```python
from build123d import *

# Parameters (mm, degrees)
BOSS_EXTRUDE1_DEPTH     = 3.556
CIRPATTERN1_COUNT       = 15
SKETCH2_W               = 7.954934775
SKETCH2_H               = 1.5875
SKETCH9_R               = 19.84375
SKETCH9_R_2             = 1.5
BOSS_EXTRUDE2_DEPTH     = 1.5875
SKETCH3_R               = 1.74625
CUT_EXTRUDE1_DEPTH      = 6.087499985
CUT_EXTRUDE1_DEPTH_BACK = 6.087499985
CIRPATTERN2_COUNT       = 4
SKETCH12_R              = 3.175
CUT_EXTRUDE2_DEPTH      = 3.175
SKETCH13_R              = 1.525
CUT_EXTRUDE4_DEPTH      = 7.99999997


with BuildPart() as part:
    # Sketch1 → Boss-Extrude1 (new body, symmetric)
    with BuildSketch(Plane(origin=(0, 0, 0), x_dir=(1, 0, 0), z_dir=(0, 1, 0))):
        with BuildLine():
            ThreePointArc((0.866466766, 6.246873729), (0.552789859, 5.752672402), (0, 5.560184675))
            ThreePointArc((0, 5.560184675), (-1.156027397, -5.438681299), (2.261530849, 5.079481453))
            ThreePointArc((2.261530849, 5.079481453), (1.834823997, 5.480167634), (1.749275672, 6.059226903))
            ThreePointArc((1.749275672, 6.059226903), (1.687548707, 6.408986287), (1.409147818, 6.629519254))
            ThreePointArc((1.409147818, 6.629519254), (1.065117112, 6.541288206), (0.866466766, 6.246873729))
        make_face()
    boss_extrude1 = extrude(amount=BOSS_EXTRUDE1_DEPTH, both=True)

    # CirPattern1: Boss-Extrude1 ×15 about axis
    cirpattern1_axis = Axis((0, 0, 0), (0, 1, 0))
    for i in range(1, CIRPATTERN1_COUNT):
        add(boss_extrude1.rotate(cirpattern1_axis, i * 360 / CIRPATTERN1_COUNT))

    # Sketch2 → Revolve3 (revolve)
    with BuildSketch(Plane(origin=(0, 0, 0), x_dir=(0, 0, -1), z_dir=(1, 0, 0))):
        with Locations((3.977467388, 4.293749985)):
            Rectangle(SKETCH2_W, SKETCH2_H)
    revolve3 = revolve(axis=Axis((0, 3.3, 0), (0, -1, 0)))

    # Mirror1: Revolve3 across plane
    add(revolve3.mirror(Plane.ZX))

    # Sketch9 → Boss-Extrude2 (add)
    with BuildSketch(Plane.XZ.offset(5.087499985)):
        Circle(SKETCH9_R)
        Circle(SKETCH9_R_2, mode=Mode.SUBTRACT)
    extrude(amount=-BOSS_EXTRUDE2_DEPTH)

    # Sketch3 → Cut-Extrude1 (cut, two sides)
    with BuildSketch(Plane(origin=(0, 0, 0), x_dir=(1, 0, 0), z_dir=(0, 1, 0))) as cut_extrude1_sk:
        with Locations((-15.5, 0)):
            Circle(SKETCH3_R)
        with Locations((0, 15.5)):
            Circle(SKETCH3_R)
        with Locations((15.5, 0)):
            Circle(SKETCH3_R)
        with Locations((0, -15.5)):
            Circle(SKETCH3_R)
    extrude(amount=CUT_EXTRUDE1_DEPTH, mode=Mode.SUBTRACT)
    extrude(cut_extrude1_sk.sketch, amount=-CUT_EXTRUDE1_DEPTH_BACK, mode=Mode.SUBTRACT)

    # Sketch6 → Cut-Revolve2 (revolve, cut)
    with BuildSketch(Plane.XY):
        Polygon((-11.8678, -3.499999985), (-15.5, -7.132199985), (-15.5, -3.499999985), align=None)
    cut_revolve2 = revolve(axis=Axis((-15.5, -5.087499985, 0), (0, 1, 0)), mode=Mode.SUBTRACT)

    # CirPattern2: Cut-Revolve2 ×4 about axis
    cirpattern2_axis = Axis((0, 0, 0), (0, 1, 0))
    for i in range(1, CIRPATTERN2_COUNT):
        add(cut_revolve2.rotate(cirpattern2_axis, i * 360 / CIRPATTERN2_COUNT), mode=Mode.SUBTRACT)

    # Sketch12 → Cut-Extrude2 (cut)
    with BuildSketch(Plane(origin=(0, 5.087499985, 0), x_dir=(1, 0, 0), z_dir=(0, 1, 0))):
        Circle(SKETCH12_R)
    extrude(amount=-CUT_EXTRUDE2_DEPTH, mode=Mode.SUBTRACT)

    # Sketch13 → Cut-Extrude4 (cut, through all)
    with BuildSketch(Plane(origin=(0, 1.912499985, 0), x_dir=(1, 0, 0), z_dir=(0, 1, 0))):
        Circle(SKETCH13_R)
    extrude(amount=-CUT_EXTRUDE4_DEPTH, mode=Mode.SUBTRACT)


solid = part.part
```
CAD build for the part. Positions are in the model's coordinates, mm. A direction names the side the tool comes from. Give positions to 0.01 mm unless a question says otherwise; leave off trailing zeros. Order: outer loops, then holes, each group sorted by start corner. A loop starts at its lowest first (then second) coordinate and runs counter-clockwise, first axis right, second up.
(1) Saw through at D-D, the plane x = 9. Give the cut face in (y, z).
(2) Mould opens along Z. For faces 1 (the flat face through (-3.4, 5.087, -0.1)), 2 (the flat face through (-0.8, 1.912, -1.5)), 3 (the cylindrical face through (18.927, -4.305, 5.961)) say: released by +Z, released by -Z, zero draft, split by the parting line, or undercut.
(3) Tool access for faces 4 (the cylindrical face through (-1.524, -1.539, -0.067)), 5 (the cylindrical face through (-0.69, 3.52, 3.1)), 6 (the flat face through (-2.3, 3.5, -5.3)): list every direction of +Z, -Z, +X, -X, +Y, -Y with a clear straight run to the whole face (end or side of a thin tool).
(4) Drill centre lines: L1, parallel to X at y = 4.2, z = 0 (3 decimals); L2, parallel to X at y = -1.5, z = 0 (3 decimals); L3, parallel to Y at x = -2, z = -5.5. Where is each one in solid material? Low to high.
(5) Saw through at A-A, the plane x = 15.5. Give the cut face in (y, z), then the cut area to 3 significant figures.
(6) Flat gauge pins, fed straight in: pin 1 (5 mm diameter, centred on x = 0, z = 0, fed in from +Y); pin 2 (4 mm diameter, centred on x = 14, z = -8, fed in from +Y); pin 3 (4 mm diameter, centred on x = -13, y = -4, fed in from +Z). Where does each tip first touch, or does it go through?
(7) Saw through at C-C, the plane z = -10. Give the cut face in (x, y).
(8) Saw through at B-B, the plane z = -15.5. Give the cut face in (x, y).
Results found:
1. outline: (-5.09, -17.69) - (-3.5, -17.69) - (-3.5, 17.69) - (-5.09, 17.69) - close
2. face 1: zero draft
2. face 2: undercut
2. face 3: split by the parting line
3. face 4: +Y, -Y
3. face 5: +Y
3. face 6: none
4. L1: x = -7.955 to -3.175, 3.175 to 7.955
4. L2: x = -5.834 to -1.525, 1.525 to 5.834
4. L3: y = -5.09 to -3.5, 3.5 to 5.09
5. outline: (-5.09, -12.39) - (-3.5, -12.39) - (-3.5, -3.63) - (-5.09, -2.04) - close; (-5.09, 2.04) - (-3.5, 3.63) - (-3.5, 12.39) - (-5.09, 12.39) - close
5. area: 30.3 mm2
6. pin 1: stops at y = 1.91
6. pin 2: stops at y = -3.5
6. pin 3: stops at z = 16.52
7. outline: (-17.14, -5.09) - (17.14, -5.09) - (17.14, -3.5) - (-17.14, -3.5) - close
8. outline: (-12.39, -5.09) - (-2.04, -5.09) - (-3.63, -3.5) - (-12.39, -3.5) - close; (2.04, -5.09) - (12.39, -5.09) - (12.39, -3.5) - (3.63, -3.5) - close
